Verification items for the finished model (mm, model axes). Face numbers are marked on the shaded views. Round coordinates to 2 decimals unless told otherwise and drop trailing zeros. Write each loop counter-clockwise with the first axis right and the second up, starting at its lowest first coordinate (ties: lowest second). Pieces come first, ordered by that corner, then holes. Notation, with made-up numbers: (86, 71) - (93, 71) arc R21 ccw to (93, 108) - close; hole circle Ø10 at (34, 60). An arc over 180 degrees is marked (long way). Answer as a JSON object with one key per item and string values. Group by question number.
1) Section check B-B (y = -13). Enter the section's corners in (x, z) (3 decimals), then the cut area to 3 significant figures.
2) Section check A-A (x = -6). Enter the section's corners in (y, z) (3 decimals).
3) Section check D-D (z = 455). Enter the section's corners in (x, y) (3 decimals), then the cut area to 3 significant figures.
4) Thickness scan on line 1 (Y direction, x = 0.5, z = 251) (3 decimals); line 2 (Y direction, x = 6.5, z = 59.5) (3 decimals). Record the ranges inside material, lowest first.
5) Section check C-C (z = 203). Enter the section's corners in (x, y) (3 decimals).
6) Mould release check, pull along X, two halves, no side actions. Record for the marked faces 1, 2 and 3: +X half, -X half, draft (parallel to the pull), parting line (faces both ways), or undercut.
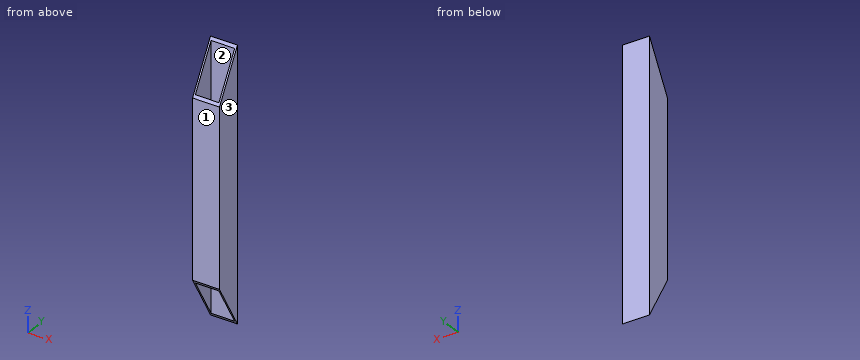
```python
from build123d import *

# Parameters (mm, degrees)
SKETCH1_W           = 50.8
SKETCH1_H           = 50.8
SKETCH1_W_2         = 44.45
SKETCH1_H_2         = 44.45
BOSS_EXTRUDE1_DEPTH = 508
CUT_EXTRUDE1_DEPTH  = 512.165139656


with BuildPart() as part:
    # Sketch1 → Boss-Extrude1 (new body)
    with BuildSketch(Plane.XY):
        Rectangle(SKETCH1_W, SKETCH1_H)
        Rectangle(SKETCH1_W_2, SKETCH1_H_2, mode=Mode.SUBTRACT)
    extrude(amount=BOSS_EXTRUDE1_DEPTH)

    # Sketch2 → Cut-Extrude1 (cut, through all)
    with BuildSketch(Plane.ZY.offset(25.4)):
        Polygon((0, 25.4), (87.988181024, -25.4), (0, -25.4), align=None)
        Polygon((508, 25.4), (420.011818975, -25.4), (508, -25.4), align=None)
    extrude(amount=-CUT_EXTRUDE1_DEPTH, mode=Mode.SUBTRACT)


solid = part.part
```
Returned:
{
 "1": {"outline": "(-25.4, 66.511) - (-22.225, 66.511) - (-22.225, 441.489) - (-25.4, 441.489) - close; (22.225, 66.511) - (25.4, 66.511) - (25.4, 441.489) - (22.225, 441.489) - close", "area": "2,380 mm2"},
 "2": {"outline": "(-25.4, 87.988) - (-22.225, 82.489) - (-22.225, 425.511) - (-25.4, 420.012) - close; (22.225, 5.499) - (25.4, 0) - (25.4, 508) - (22.225, 502.501) - close"},
 "3": {"outline": "(-25.4, -5.2) - (-22.225, -5.2) - (-22.225, 22.225) - (22.225, 22.225) - (22.225, -5.2) - (25.4, -5.2) - (25.4, 25.4) - (-25.4, 25.4) - close", "area": "335 mm2"},
 "4": {"line 1": "-25.4 to -22.225, 22.225 to 25.4", "line 2": "22.225 to 25.4"},
 "5": {"outline": "(-25.4, -25.4) - (25.4, -25.4) - (25.4, 25.4) - (-25.4, 25.4) - close; hole (-22.225, -22.225) - (22.225, -22.225) - (22.225, 22.225) - (-22.225, 22.225) - close"},
 "6": {"face 1": "draft", "face 2": "undercut", "face 3": "+X half"}
}
